Geometry check sheet. Reference: the model listing, model coordinates, mm. Face numbers are marked on the shaded views. A direction names the side the tool comes from. Round coordinates to 2 decimals unless told otherwise and drop trailing zeros. Loops run counter-clockwise (first coordinate to the right, second up) from the corner with the lowest first, then second, coordinate; pieces in that order, holes last. Notation, with made-up numbers: M 9,14.5 L 34,14.5 A19 ccw 34,40.5 Z; hole C 81.5,51.5 d6. An arc over 180 degrees is marked long. Write item = value, one per line.
from build123d import *

# Parameters (mm, degrees)
F0_R     = 12.7
F1_DEPTH = 19.05
F2_R     = 11.90625
F3_DEPTH = 17.78
F5_DEPTH = 3.175


with BuildPart() as f1:
    # F0 (on Top) → F1 (new body)
    with BuildSketch(Plane.XY):
        with Locations((0, 0.932285)):
            Circle(F0_R)
    extrude(amount=F1_DEPTH)

    # F2 (on face) → F3 (cut)
    with BuildSketch(Plane.XY.offset(19.05)):
        with Locations((0, 0.932285)):
            Circle(F2_R)
    extrude(amount=-F3_DEPTH, mode=Mode.SUBTRACT)

    # F4 (on Right) → F5 (join, symmetric)
    with BuildSketch(Plane.YZ):
        Polygon((12.734854, 4.566981), (12.734854, 0), (54.188989, 0), (54.188989, 4.566981), (54.188989, 15.281822), (50.500277, 15.281822), (50.500277, 4.566981), (45.230679, 4.566981), (45.230679, 15.106169), (41.717619, 15.106169), (41.717619, 4.566981), align=None)
    extrude(amount=F5_DEPTH, both=True)


solid = f1.part
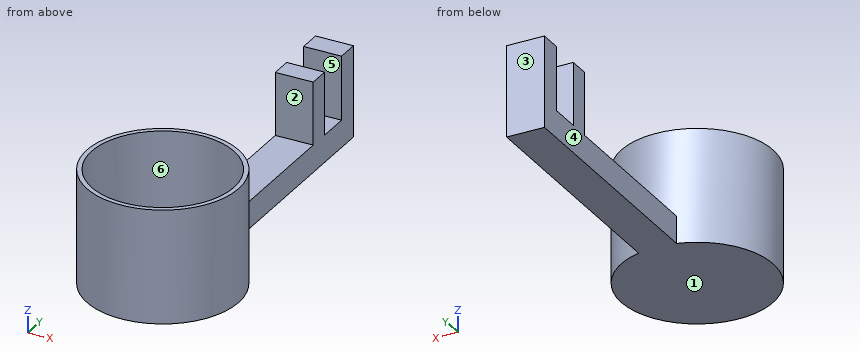
(1) Sectioned sample at C-C on x = 0. Record the cut outline in (y, z), then the cut area to 3 significant figures.
Result set:
outline = M -11.77,0 L 54.19,0 L 54.19,15.28 L 50.5,15.28 L 50.5,4.57 L 45.23,4.57 L 45.23,15.11 L 41.72,15.11 L 41.72,4.57 L 13.63,4.57 L 13.63,19.05 L 12.84,19.05 L 12.84,4.57 L 12.73,4.57 L 12.73,1.27 L -10.97,1.27 L -10.97,19.05 L -11.77,19.05 Z
area = 323 mm2
(2) Release check for a two-part mould opening along Y. For the marked faces 1, 2 and 3 record: released by +Y, released by -Y, zero draft, split by the parting line, or undercut.
Result set:
face_1 = zero draft
face_2 = undercut
face_3 = released by +Y
(3) Depth check by flat-ended pin: pin 1 Ø1.5 at (x, z) = (6.5, 4) entering from +Y; pin 2 Ø12 at (x, y) = (1, -1) entering from +Z; pin 3 Ø1.9 at (x, y) = (-1.5, 20.5) entering from +Z. Enter the tip coordinate at first touch or a pass-through.
Result set:
pin_1 = 12.26
pin_2 = 1.27
pin_3 = 4.57
(4) Sectioned sample at A-A on z = 3. Record the cut outline in (x, y) (1 decimal), then the cut area to 3 significant figures.
Result set:
outline = M -3.2,13.2 A12.7 ccw long 3.2,13.2 L 3.2,54.2 L -3.2,54.2 Z; hole M -1.6,12.7 A11.9 ccw long 1.6,12.7 Z
area = 320 mm2
(5) Tool access check on the marked faces 4, 5 and 6. Record the directions out of +Z, -Z, +X, -X, +Y, -Y that give a thin tool (end or side, any length) a straight path to the whole face; none if there is none.
Result set:
face_4 = +Z, -Z, -X, +Y
face_5 = +Z, +X, -X
face_6 = +Z
(6) Material ranges on line 1 along Y through (x, z) = (0, 12.25); line 2 along Y through (x, z) = (-3, 8); line 3 along Y through (x, z) = (5.75, 18.25), recorded low to high. Write a range as from..to.
Result set:
line_1 = -11.77..-10.97, 12.84..13.63, 41.72..45.23, 50.5..54.19
line_2 = -11.41..-10.59, 12.45..13.27, 41.72..45.23, 50.5..54.19
line_3 = -10.39..-9.49, 11.36..12.26
(7) Sectioned sample at D-D on y = 6.5. Record the cut outline in (x, z).
Result set:
outline = M -11.41,0 L 11.41,0 L 11.41,19.05 L 10.52,19.05 L 10.52,1.27 L -10.52,1.27 L -10.52,19.05 L -11.41,19.05 Z
(8) Sectioned sample at B-B on z = 10. Record the cut outline in (x, y) (1 decimal).
Result set:
outline = C 0,0.9 d25.4; M -3.2,41.7 L 3.2,41.7 L 3.2,45.2 L -3.2,45.2 Z; M -3.2,50.5 L 3.2,50.5 L 3.2,54.2 L -3.2,54.2 Z; hole C 0,0.9 d23.8
